Geometry check sheet. Reference: the model listing, model coordinates, mm. A direction names the side the tool comes from. Give positions to 0.01 mm unless a question says otherwise; leave off trailing zeros. Order: outer loops, then holes, each group sorted by start corner. A loop starts at its lowest first (then second) coordinate and runs counter-clockwise, first axis right, second up.
from build123d import *

# Parameters (mm, degrees)
BOSS_EXTRUDE1_DEPTH = 3.175
SKETCH3_W           = 7.62
SKETCH3_H           = 7.62
BOSS_EXTRUDE2_DEPTH = 6.35
CUT_EXTRUDE1_REACH  = 66.96
SKETCH5_R           = 1.5875
SKETCH6_R           = 1.27
BOSS_EXTRUDE3_DEPTH = 3.302
SKETCH9_R           = 1.651
CUT_EXTRUDE3_DEPTH  = 3.175


with BuildPart() as part:
    # Sketch2 → Boss-Extrude1 (new body)
    with BuildSketch(Plane(origin=(0, 0, 0), x_dir=(1, 0, 0), z_dir=(0, 1, 0))):
        with BuildLine():
            Line((3.81, 45.72), (3.81, -45.72))
            ThreePointArc((3.81, -45.72), (1.344074772, -49.285047406), (-2.861686618, -48.235322981))
            Line((-2.861686618, -48.235322981), (-41.91, -3.81))
            Line((-41.91, -3.81), (-34.29, -3.81))
            Line((-34.29, -3.81), (-3.81, -38.487140373))
            Line((-3.81, -38.487140373), (-3.81, 38.487140373))
            Line((-3.81, 38.487140373), (-34.29, 3.81))
            Line((-34.29, 3.81), (-41.91, 3.81))
            Line((-41.91, 3.81), (-2.861686618, 48.235322981))
            ThreePointArc((-2.861686618, 48.235322981), (1.344074772, 49.285047406), (3.81, 45.72))
        make_face()
    extrude(amount=BOSS_EXTRUDE1_DEPTH)

    # Sketch3 → Boss-Extrude2 (add)
    with BuildSketch(Plane(origin=(0, 0, 0), x_dir=(1, 0, 0), z_dir=(0, 1, 0))):
        with Locations((-38.1, 0)):
            Rectangle(SKETCH3_W, SKETCH3_H)
    extrude(amount=BOSS_EXTRUDE2_DEPTH)

    # Sketch5 → Cut-Extrude1 (cut, up to next)
    with BuildSketch(Plane(origin=(0, 3.175, 0), x_dir=(1, 0, 0), z_dir=(0, 1, 0)), mode=Mode.PRIVATE) as cut_extrude1_sk1:
        with Locations(Location((0, 0, 0), (0, 0, 270))):
            Circle(SKETCH5_R)
    cut_extrude1_tool1 = extrude(cut_extrude1_sk1.sketch, amount=-CUT_EXTRUDE1_REACH, mode=Mode.PRIVATE) & part.part
    add(cut_extrude1_tool1.solids().sort_by_distance((0, 3.175, 0))[0], mode=Mode.SUBTRACT)

    # Sketch6 → Boss-Extrude3 (add)
    with BuildSketch(Plane(origin=(0, 3.175, 0), x_dir=(1, 0, 0), z_dir=(0, 1, 0))):
        with Locations(Location((0, 45.72, 0), (0, 0, 90))):
            Circle(SKETCH6_R)
        with Locations(Location((0, -45.72, 0), (0, 0, 90))):
            Circle(SKETCH6_R)
    extrude(amount=BOSS_EXTRUDE3_DEPTH)

    # Sketch9 → Cut-Extrude3 (cut)
    with BuildSketch(Plane.ZY.offset(41.91)):
        with Locations((0, 3.175)):
            Circle(SKETCH9_R)
    extrude(amount=-CUT_EXTRUDE3_DEPTH, mode=Mode.SUBTRACT)


solid = part.part
Item 1: Gauge pin test, flat ends, axial feed: pin 1 (3 mm diameter, centred on x = -3.5, y = 3.5, fed in from +Z); pin 2 (1.9 mm diameter, centred on y = 4.5, z = 1.5, fed in from +X); pin 3 (1.7 mm diameter, centred on y = 2.5, z = 0, fed in from -X) (3 decimals). Record the tip position at first contact, or that the pin passes through.
Reported:
pin 1: stops at z = 48.94
pin 2: stops at x = -34.29
pin 3: stops at x = -38.735
Item 2: Scan lines: L1, parallel to X at y = 2.4, z = 0 (1 decimal); L2, parallel to X at y = 0.75, z = 0; L3, parallel to X at y = 3, z = 2.5. Record each from-to range of solid material in increasing order.
Reported:
L1: x = -38.7 to -34.3, -3.8 to -1.6, 1.6 to 3.8
L2: x = -41.91 to -34.29, -3.81 to -1.59, 1.59 to 3.81
L3: x = -41.91 to -34.29, -3.81 to 3.81
Item 3: Draft check along X on faces 6 (the flat face through (-3.81, 2, 1)), 7 (the cylindrical face through (-40.345, 4.812, -0.215)), 8 (the flat face through (3.81, 2, -1)). Enter one of: released by +X, released by -X, zero draft, split by the parting line, or undercut.
Reported:
face 6: undercut
face 7: zero draft
face 8: released by +X
Item 4: Sectioned sample at B-B (z = 0). Give the number of separate pieces and of enclosed holes in the cut face, and give its area (3 significant figures).
Reported:
separate pieces: 3
enclosed holes: 0
area: 52.0 mm2
Item 5: Sectioned sample at D-D (x = -16.5). Enter the section's corners in (y, z) (3 decimals), and give its area (4 significant figures).
Reported:
outline: (0, -32.719) - (3.175, -32.719) - (3.175, -24.05) - (0, -24.05) - close; (0, 24.05) - (3.175, 24.05) - (3.175, 32.719) - (0, 32.719) - close
area: 55.05 mm2
Item 6: Set-up check for faces 1 (the flat face through (-38, 5, 3.81)), 2 (the flat face through (-34.29, 3, 0)), 3 (the cylindrical face through (0.49, 4.8, 44.55)), 4 (the flat face through (-38.735, 3, 0)), 5 (the cylindrical face through (1.3, 1.6, -49.3)): record each of +Z, -Z, +X, -X, +Y, -Y from which the full face is reachable in a straight line by a thin tool's end or side.
Reported:
face 1: +Z, +X, -X, +Y
face 2: +Y, -Y
face 3: +Y
face 4: -X
face 5: -Z, +Y, -Y
Item 7: Sectioned sample at C-C (z = -15). Enter the section's corners in (x, y) (3 decimals).
Reported:
outline: (-32.074, 0) - (-24.454, 0) - (-24.454, 3.175) - (-32.074, 3.175) - close; (-3.81, 0) - (3.81, 0) - (3.81, 3.175) - (-3.81, 3.175) - close
